```python
from build123d import *

# Parameters (mm, degrees)
F0_W     = 228.6
F0_H     = 152.297022
F1_DEPTH = 50.8
F3_DEPTH = 50.8


with BuildPart() as f1:
    # F0 (on Front) → F1 (new body)
    with BuildSketch(Plane.XZ):
        with Locations((-3.682856, -7.733995)):
            Rectangle(F0_W, F0_H)
    extrude(amount=F1_DEPTH)

    # F2 (on Front) → F3 (join, symmetric)
    with BuildSketch(Plane.XZ):
        Polygon((-15.677309, -7.330912), (-117.277309, -7.330912), (-117.277309, -83.527267), (60.522691, -83.527267), (60.522691, 68.872733), (-15.677309, 68.872733), align=None)
    extrude(amount=F3_DEPTH, both=True)


solid = f1.part
```
Design review of the part built by this model. Coordinates are the model's own, in mm. A direction names the side the tool comes from. Coordinates: 2 decimals unless noted, no trailing zeros. Loops run counter-clockwise (first coordinate to the right, second up) from the corner with the lowest first, then second, coordinate; pieces in that order, holes last. Notation, with made-up numbers: M 15,-5 L 38,-5 A10 cw 38,8 Z; hole C -28.5,64 d2. An arc over 180 degrees is marked long. One line per question, with ' | ' between items.
(1) We need section B-B (z = 37.5). Give the boundary of the cut face in (x, y).
Filled in:
outline: M -117.98,-50.8 L 110.62,-50.8 L 110.62,0 L 60.52,0 L 60.52,50.8 L -15.68,50.8 L -15.68,0 L -117.98,0 Z
(2) We need section C-C (y = 28). Give the boundary of the cut face in (x, z).
Filled in:
outline: M -117.28,-83.53 L 60.52,-83.53 L 60.52,68.87 L -15.68,68.87 L -15.68,-7.33 L -117.28,-7.33 Z
(3) We need section D-D (x = 95). Give the boundary of the cut face in (y, z), and give its area (3 significant figures).
Filled in:
outline: M -50.8,-83.88 L 0,-83.88 L 0,68.41 L -50.8,68.41 Z | area: 7,740 mm^2
(4) Machinability: for faces 1 (the face through (-30, 25, -83.527)), 2 (the face through (-68, -25, 68.415)), 3 (the face through (85, -25, 68.415)), 4 (the face through (-66, 25, -7.331)), 5 (the face through (-117.277, 25, -45)), which of the approach directions +Z, -Z, +X, -X, +Y, -Y give a long, thin tool a straight path to every point of the face, cutting with its end or side? Answer none if there is none.
Filled in:
face 1: -Z, +X, -X, +Y | face 2: +Z, -X, +Y, -Y | face 3: +Z, +X, +Y, -Y | face 4: +Z, -X, +Y | face 5: +Z, -Z, -X, +Y
(5) We need section A-A (x = -100.5). Give the boundary of the cut face in (y, z), and give its area (3 significant figures).
Filled in:
outline: M -50.8,-83.88 L 0,-83.88 L 0,-83.53 L 50.8,-83.53 L 50.8,-7.33 L 0,-7.33 L 0,68.41 L -50.8,68.41 Z | area: 11,600 mm^2
(6) Wall thickness on probe 1 along Z at (x, y) = (18, 2); probe 2 along X at (y, z) = (5.5, 9); probe 3 along Z at (x, y) = (-89, -12.5): over which ranges is each line inside the solid? List them lowest first.
Filled in:
probe 1: z = -83.53 to 68.87 | probe 2: x = -15.68 to 60.52 | probe 3: z = -83.88 to 68.41
(7) For pin 1 Ø2 at (y, z) = (27, -36) entering from -X; pin 2 Ø10 at (y, z) = (31, 17.5) entering from +X; pin 3 Ø15 at (x, y) = (-48, -13) entering from +Z, all flat-tipped, find the tip position at first contact; note any pin that passes through.
Filled in:
pin 1: stops at x = -117.28 | pin 2: stops at x = 60.52 | pin 3: stops at z = 68.41
